Could you check a few things on this model? Use its own coordinates, in mm. Face numbers are marked on the shaded views. A direction names the side the tool comes from. Give positions to 0.01 mm unless a question says otherwise; leave off trailing zeros. Order: outer loops, then holes, each group sorted by start corner. A loop starts at its lowest first (then second) coordinate and runs counter-clockwise, first axis right, second up. Notation, with made-up numbers: (0.25, 76) -> (35.25, 76) arc R22 cw to (35.25, 112) -> close; hole circle Ø3 at (7, 6). An arc over 180 degrees is marked (long way). Use one line per item in the form item = value. Start each with the question number.
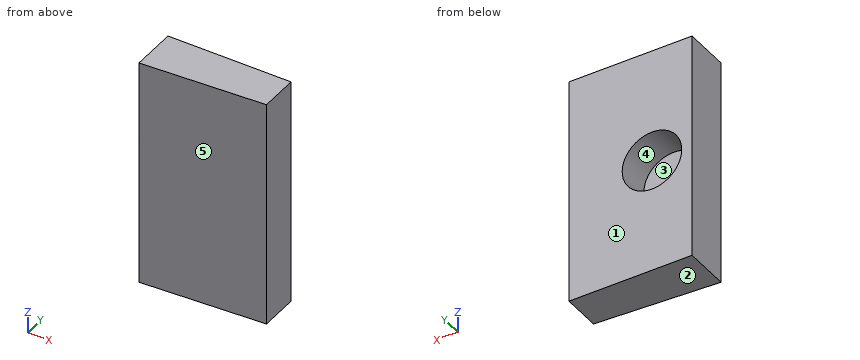
Autodesk Inventor part; units mm, degrees
ref_plane "YZ Plane" through (0, 0, 0) normal (1, 0, 0) x (0, 1, 0)
ref_plane "XZ Plane" through (0, 0, 0) normal (0, 1, 0) x (-1, 0, 0)
ref_plane "XY Plane" through (0, 0, 0) normal (0, 0, 1) x (1, 0, 0)
sketch "Sketch1" plane through (0, 0, 0) normal (0, 1, 0) x (-1, 0, 0)
  line L0 (0, 0) -> (35, 0)
  line L1 (35, 0) -> (35, -20)
  line L2 (35, -20) -> (0, -20)
  line L3 (0, -20) -> (0, 0)
  dimension "d0" = 35
  dimension "d1" = 20
extrude "Extrusion1" add sketch "Sketch1" along normal blind 2
sketch "Sketch2" plane through (0, 2, 0) normal (0, 1, 0) x (1, 0, 0)
  line L0 (-35, 20) -> (-35, 0)
  line L1 (-35, 10) -> (-31.5, 10)
  circle A0 centre (-31.5, 10) radius 2.6
  point P0 (0, 0)
  dimension "d4" = 3.5
  dimension "d5" = 5.2
extrude "Extrusion2" cut sketch "Sketch2" against normal blind 2
sketch "Sketch3" plane through (-35, 0, 0) normal (0, 0, 1) x (1, 0, 0)
  line L0 (35, 0) -> (0, 0)
  line L1 (0, 0) -> (0, -2)
  line L2 (0, -2) -> (35, 0)
  dimension "d8" = 2
extrude "Extrusion3" add sketch "Sketch3" against normal up to surface (20 mm away)
sketch "Sketch4" plane through (0, 2, 0) normal (1, 0, 0) x (0, 0, -1)
  line L0 (0, -2) -> (20, -2)
  line L1 (0, -2) -> (20, -2)
  line L2 (20, -2) -> (20, 6.5769)
  line L3 (20, 6.5769) -> (0, 6.5769)
  line L4 (0, 6.5769) -> (0, -2)
extrude "Extrusion4" cut sketch "Sketch4" against normal blind 23.75
sketch "Sketch5" plane through (0, 0, 0) normal (0, 1, 0) x (1, 0, 0)
  line L0 (-23.75, 20) -> (-35, 20)
  line L1 (-23.75, 20) -> (0, 20)
  line L2 (0, 20) -> (0, 0)
  line L3 (0, 0) -> (-23.75, 0)
  line L4 (-23.75, 0) -> (-23.75, 20)
extrude "Extrusion5" cut sketch "Sketch5" against normal through all
sketch "Sketch6" plane through (-23.75, 2, 0) normal (1, 0, 0) x (0, 0, -1)
  line L0 (20, -4) -> (20, 0)
  line L1 (20, 0) -> (0, 0)
  line L2 (0, 0) -> (0, -8.1158)
  line L3 (0, -8.1158) -> (20, -8.1158)
  line L4 (20, -8.1158) -> (20, 0)
  point P0 (0, -2)
extrude "Extrusion6" cut sketch "Sketch6" against normal blind 0.5
sketch "Sketch7" plane through (-31.5, 0, -10) normal (0, 1, 0) x (1, 0, 0)
  circle A0 centre (0, 0) radius 2.6
  point P0 (31.5, -10)
  dimension "d19" = 5.2
extrude "Extrusion7" cut sketch "Sketch7" against normal blind 1
properties part number "opaska_test"
(1) Which directions (+Z, -Z, +X, -X, +Y, -Y) give clear straight access to the entire face, cutting with the end or side of a thin tool? Please do the marked faces 4 and 5.
(2) Please list where these lines run through material, in increasing order: probe 1 along Z at (x, y) = (-31.5, 0.55); probe 2 along X at (y, z) = (0.1, -10); probe 3 along Z at (x, y) = (-33, 1.7).
(3) Imagine slicing it at C-C (x = -31.5). Write out the boundary of the cut face in (y, z), plus the area to 3 significant figures.
(4) I'm going to push a flat-ended pin straight in: pin 1 Ø4 at (x, z) = (-32, -9) entering from +Y. Where does the tip first touch, or does it pass through?
(5) Imagine slicing it at B-B (y = 0.85). Write out the boundary of the cut face in (x, z).
(6) We'd pull the mould along Z, two halves only. Please class the marked faces 1, 2 and 3: pulls with the +Z half, pulls with the -Z half, needs draft (parallel to the pull), parting line crosses it, or undercut.
(7) Imagine slicing it at A-A (z = -10). Write out the boundary of the cut face in (x, y), plus the area to 3 significant figures.
(8) Imagine slicing it at D-D (y = -1.6). Write out the boundary of the cut face in (x, z), plus the area to 3 significant figures.
Calculated:
q1.face_4 = +Y
q1.face_5 = +Z, -Z, +X, -Y
q2.probe_1 = -20 to -12.6, -7.4 to 0
q2.probe_2 = -35 to -34.1, -28.9 to -24.25
q2.probe_3 = -20 to -12.12, -7.88 to 0
q3.outline = (-1.8, -20) -> (2, -20) -> (2, -12.6) -> (-1, -12.6) -> (-1, -7.4) -> (2, -7.4) -> (2, 0) -> (-1.8, 0) -> close
q3.area = 60.4 mm2
q4.pin_1 = 2
q5.outline = (-35, -20) -> (-24.25, -20) -> (-24.25, 0) -> (-35, 0) -> close; hole circle Ø5.2 at (-31.5, -10)
q6.face_1 = needs draft
q6.face_2 = pulls with the -Z half
q6.face_3 = undercut
q7.outline = (-35, -2) -> (-24.25, -1.39) -> (-24.25, 2) -> (-28.9, 2) -> (-28.9, -1) -> (-34.1, -1) -> (-34.1, 2) -> (-35, 2) -> close
q7.area = 24.1 mm2
q8.outline = (-35, -20) -> (-28, -20) -> (-28, 0) -> (-35, 0) -> close
q8.area = 140 mm2
